Input: part model. Units: mm. Frame: model coordinates. Face numbers are marked on the shaded views. A direction names the side the tool comes from. Give positions to 0.01 mm unless a question says otherwise; leave off trailing zeros. Loops run counter-clockwise (first coordinate to the right, second up) from the corner with the lowest first, then second, coordinate; pieces in that order, holes last. Notation, with made-up numbers: (81.25, 52) - (129.25, 52) arc R21 ccw to (129.25, 78) - close; hole circle Ø8 at (-13, 48.5). An arc over 180 degrees is marked (long way). Answer as a JSON object with one key per item and string values.
from build123d import *

# Parameters (mm, degrees)
EXTRUDE_355_DEPTH                 = 200
CUT_EXTRUDE_718_REACH             = 237.213
SKETCH_2_W                        = 13
SKETCH_2_H                        = 80
CUT_EXTRUDE_718_DIRECTION_2_DEPTH = 236.212669727
SKETCH_3_W                        = 10
SKETCH_3_H                        = 80
CUT_EXTRUDE_1071_DEPTH            = 5


with BuildPart() as part:
    # Эскиз1 → Extrude 355 (new body)
    with BuildSketch(Plane.XY):
        with BuildLine():
            Line((-45, -40), (-45, 40))
            ThreePointArc((-45, 40), (0, 85), (45, 40))
            Line((45, 40), (45, -40))
            ThreePointArc((45, -40), (0, -85), (-45, -40))
        make_face()
        with BuildLine():
            Line((-40, -40), (-40, 40))
            ThreePointArc((-40, 40), (0, 80), (40, 40))
            Line((40, 40), (40, -40))
            ThreePointArc((40, -40), (0, -80), (-40, -40))
        make_face(mode=Mode.SUBTRACT)
    extrude(amount=EXTRUDE_355_DEPTH)

    # Cut-Extrude 718: up to this face of the body (flat: up to its plane)
    cut_extrude_718_end = Plane(part.part.faces().sort_by_distance((-40, 0, 100))[0])
    # Эскиз2 → Cut-Extrude 718 (cut, up to the picked face)
    with BuildSketch(Plane.ZY.offset(45), mode=Mode.PRIVATE) as cut_extrude_718_sk1:
        with Locations((36.5, 0)):
            Rectangle(SKETCH_2_W, SKETCH_2_H)
    cut_extrude_718_tool1 = split(extrude(cut_extrude_718_sk1.sketch, amount=-CUT_EXTRUDE_718_REACH, mode=Mode.PRIVATE), bisect_by=cut_extrude_718_end, keep=Keep.BOTH, mode=Mode.PRIVATE)
    add(cut_extrude_718_tool1.solids().sort_by(Axis((-45, 0, 36.5), (1, 0, 0)))[0], mode=Mode.SUBTRACT)

    # Эскиз2 → Cut-Extrude 718 direction 2 (cut)
    with BuildSketch(Plane.ZY.offset(45)):
        with Locations((36.5, 0)):
            Rectangle(SKETCH_2_W, SKETCH_2_H)
    extrude(amount=CUT_EXTRUDE_718_DIRECTION_2_DEPTH, mode=Mode.SUBTRACT)

    # Эскиз3 → Cut-Extrude 1071 (cut)
    with BuildSketch(Plane.ZY.offset(45)):
        with Locations((165, 0)):
            Rectangle(SKETCH_3_W, SKETCH_3_H)
    extrude(amount=-CUT_EXTRUDE_1071_DEPTH, mode=Mode.SUBTRACT)


solid = part.part
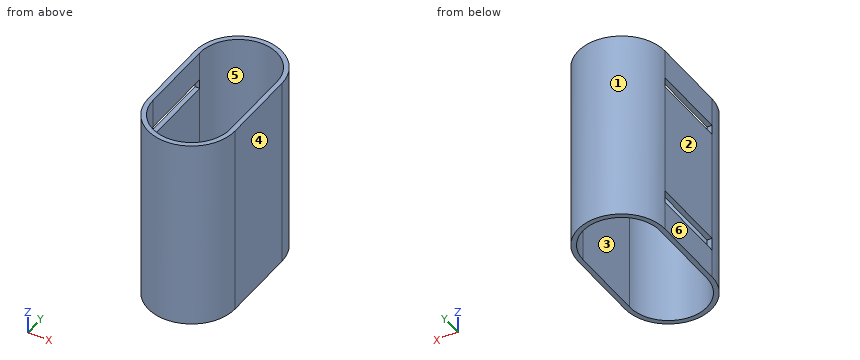
Item 1: Material intervals for line 1 (X direction, y = -7, z = 43.5); line 2 (Y direction, x = -18.5, z = 104.5); line 3 (Y direction, x = 10, z = 170), sorted ascending. Write a range as [from, to].
Geometry check:
{"line 1": "x = [-45, -40], [40, 45]", "line 2": "y = [-81.02, -75.46], [75.46, 81.02]", "line 3": "y = [-83.87, -78.73], [78.73, 83.87]"}
Item 2: Cut plane C-C (y = -34). Return loops of the section in (x, z), then the cut area to 4 significant figures.
Geometry check:
{"outline": "(-45, 0) - (-40, 0) - (-40, 30) - (-45, 30) - close; (-45, 43) - (-40, 43) - (-40, 160) - (-45, 160) - close; (-45, 170) - (-40, 170) - (-40, 200) - (-45, 200) - close; (40, 0) - (45, 0) - (45, 200) - (40, 200) - close", "area": "1,885 mm2"}
Item 3: Cut plane A-A (x = 0). Return loops of the section in (y, z), then the cut area to 3 significant figures.
Geometry check:
{"outline": "(-85, 0) - (-80, 0) - (-80, 200) - (-85, 200) - close; (80, 0) - (85, 0) - (85, 200) - (80, 200) - close", "area": "2,000 mm2"}
Item 4: Cut plane D-D (y = -52.5). Return loops of the section in (x, z).
Geometry check:
{"outline": "(-43.23, 0) - (-38, 0) - (-38, 200) - (-43.23, 200) - close; (38, 0) - (43.23, 0) - (43.23, 200) - (38, 200) - close"}
Item 5: Mould query, pull axis X, two halves, no side actions, for the marked faces 1, 2, 3 and 4. Classes: released by +X, released by -X, zero draft, split by the parting line, or undercut.
Geometry check:
{"face 1": "split by the parting line", "face 2": "released by -X", "face 3": "undercut", "face 4": "released by +X"}
Item 6: Contact query for flat-ended pins moving along their axis: P1, Ø5.5, axis at x = -41.5, y = 15, coming from the -Z side; P2, Ø10, axis at y = -50.5, z = 22.5, coming from the +X side; P3, Ø4, axis at x = -43.5, z = 37, coming from the -Y side; P4, Ø5.5, axis at x = -42, z = 39, coming from the +Y side. Output: stop coordinate, or through.
Geometry check:
{"P1": "stops at z = 0", "P2": "stops at x = 44.66", "P3": "stops at y = -57.4", "P4": "stops at y = 62.01"}
Item 7: Access query for the marked faces 5 and 6. Directions: +Z, -Z, +X, -X, +Y, -Y. A direction counts if a zero-diameter tool reaches every point of the face in a straight line with its end or side. Return the directions, or none.
Geometry check:
{"face 5": "+Z, -Z", "face 6": "+Z, -Z, -X, +Y, -Y"}
Item 8: Cut plane B-B (z = 114). Return loops of the section in (x, y).
Geometry check:
{"outline": "(-45, -40) arc R45 ccw to (45, -40) - (45, 40) arc R45 ccw to (-45, 40) - close; hole (-40, -40) arc R40 ccw to (40, -40) - (40, 40) arc R40 ccw to (-40, 40) - close"}
